Design review of the part built by this model. Coordinates are the model's own, in mm. Face numbers are marked on the shaded views. Coordinates: 2 decimals unless noted, no trailing zeros. Loops run counter-clockwise (first coordinate to the right, second up) from the corner with the lowest first, then second, coordinate; pieces in that order, holes last. Notation, with made-up numbers: (-36.5, -7.75) -> (-24.5, -7.75) arc R23 cw to (-24.5, 16.25) -> close; hole circle Ø5 at (43, 23). An arc over 180 degrees is marked (long way). One line per item, written item: value. Start each with the question number.
1. For probe 1 along Y at (x, z) = (1, 25.5); probe 2 along X at (y, z) = (-35.5, 10); probe 3 along X at (y, z) = (-32.5, 34.5), list the stretches that pass through material, from the lowest coordinate up.
2. Draft analysis for pull direction Y (two halves, no side actions). For the marked faces 1, 2, 3 and 4, state which applies: pulls with the +Y half, pulls with the -Y half, needs draft (parallel to the pull), parting line crosses it, or undercut.
3. Add section C-C on z = 27.5. Write out the cut boundary in (x, y), plus the area to 3 significant figures.
4. Add section B-B on y = -9.5. Write out the cut boundary in (x, z), plus the area to 3 significant figures.
5. Insertion check: pin 1 (10 mm diameter, centred on y = -22.5, z = 16, fed in from +X). The pin has a flat end and moves straight along its axis. Give the tip position at first contact, or say it passes through.
6. Add section A-A on x = 0. Write out the cut boundary in (y, z), plus the area to 3 significant figures.
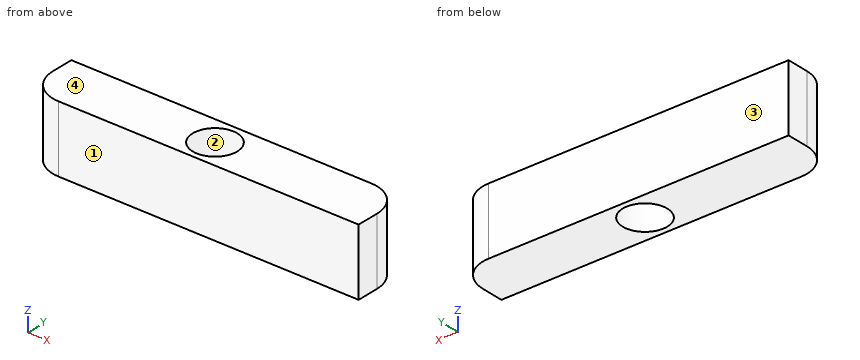
```python
from build123d import *

# Parameters (mm, degrees)
F0_W     = 300
F0_H     = 50
F0_R     = 20
F1_DEPTH = 60
F2_R     = 30


with BuildPart() as f1:
    # F0 (on Top) → F1 (new body)
    with BuildSketch(Plane.XY):
        with Locations((0, -24.096213)):
            Rectangle(F0_W, F0_H)
        with Locations((0, -24.096213)):
            Circle(F0_R, mode=Mode.SUBTRACT)
    extrude(amount=F1_DEPTH)

    # F2
    f2_edges = [f1.edges().sort_by_distance(p)[0] for p in [
        (-150, -49.096213, 30),
        (150, 0.903787, 30),
    ]]
    fillet(f2_edges, radius=F2_R)


solid = f1.part
```
Worked answers:
1. probe 1: y = -49.1 to -44.07, -4.12 to 0.9
1. probe 2: x = -145.12 to -16.43, 16.43 to 150
1. probe 3: x = -146.84 to -18.15, 18.15 to 150
2. face 1: pulls with the -Y half
2. face 2: undercut
2. face 3: pulls with the +Y half
2. face 4: needs draft
3. outline: (-150, -19.1) arc R30 ccw to (-120, -49.1) -> (150, -49.1) -> (150, -29.1) arc R30 ccw to (120, 0.9) -> (-150, 0.9) -> close; hole circle Ø40 at (0, -24.1)
3. area: 13,400 mm²
4. outline: (-150, 0) -> (-13.67, 0) -> (-13.67, 60) -> (-150, 60) -> close; (13.67, 0) -> (142.72, 0) -> (142.72, 60) -> (13.67, 60) -> close
4. area: 15,900 mm²
5. pin 1: stops at x = 149.96
6. outline: (-49.1, 0) -> (-44.1, 0) -> (-44.1, 60) -> (-49.1, 60) -> close; (-4.1, 0) -> (0.9, 0) -> (0.9, 60) -> (-4.1, 60) -> close
6. area: 600 mm²
